Autodesk Inventor part; units mm, degrees
ref_plane "Work Plane1" through (0, 0, -15) normal (0, 0, 1) x (1, 0, 0)
ref_plane "YZ Plane" through (0, 0, 0) normal (1, 0, 0) x (0, 1, 0)
ref_plane "XZ Plane" through (0, 0, 0) normal (0, 1, 0) x (-1, 0, 0)
sketch "Sketch1" plane through (0, 0, 0) normal (0, 0, 1) x (1, 0, 0)
  line L0 (0, 0) -> (25, 0)
  line L1 (25, 0) -> (25, 40)
  line L2 (25, 40) -> (0, 40)
  line L3 (0, 40) -> (0, 0)
  dimension "d1" = 25
  dimension "d2" = 40
  dimension "d3" = 25
extrude "Extrusion1" add sketch "Sketch1" against normal blind 30
sketch "Sketch2" plane through (25, 0, 0) normal (1, 0, 0) x (0, 0, -1)
  line L0 (0, 0) -> (30, 0)
  circle A0 centre (15, 6.56) radius 2.46
extrude "Extrusion2" cut sketch "Sketch2" against normal blind 30
sketch "Sketch3" plane through (0, 0, 0) normal (-1, 0, 0) x (0, 0, 1)
  line L0 (0, 0) -> (-30, 0)
  line L1 (-25.05, 0) -> (-4.95, 0)
  line L2 (-4.95, 0) -> (-4.95, 33.12)
  line L3 (-4.95, 33.12) -> (-25.05, 33.12)
  line L4 (-25.05, 33.12) -> (-25.05, 0)
  dimension "d11" = 20.1
extrude "Extrusion3" cut sketch "Sketch3" against normal blind 20
sketch "Sketch4" plane through (0, 0, 0) normal (0, -1, 0) x (1, 0, 0)
  line L0 (20, -4.95) -> (20, -25.05)
  line L1 (20, -15) -> (25, -15)
  line L2 (25, 0) -> (25, -30)
  line L3 (20, -8.025) -> (25, -8.025)
  line L4 (25, -8.025) -> (25, -21.975)
  line L5 (25, -21.975) -> (20, -21.975)
  line L6 (20, -21.975) -> (20, -8.025)
  line L7 (20, -8.025) -> (25, -21.975) construction
  line L8 (25, -8.025) -> (20, -21.975) construction
  line L9 (25, -12.54) -> (25, -17.46)
  point P0 (0, 0)
  point P1 (22.5, -15)
  dimension "d14" = 13.95
extrude "Extrusion4" add sketch "Sketch4" along normal blind 15
sketch "Sketch5" plane through (20, 0, 0) normal (-1, 0, 0) x (0, 0, 1)
  circle A0 centre (-15, 6.56) radius 2.46
  circle A1 centre (-15, 6.56) radius 4.7025
  circle A2 centre (-15, 6.56) radius 2.46
  circle A3 centre (-15, 6.56) radius 2.46
  point P0 (0, 0)
  dimension "d17" = 9.405
extrude "Extrusion5" cut sketch "Sketch5" against normal blind 2.1
sketch "Sketch6" plane through (25, 0, 0) normal (1, 0, 0) x (0, 0, -1)
  circle A0 centre (15, 6.56) radius 4.7025
  line L0 (15, 6.56) -> (15, 23.56)
  circle A1 centre (15, 23.56) radius 2.46
  point P0 (0, 0)
  dimension "d20" = 17
  dimension "d21" = 4.92
extrude "Extrusion6" cut sketch "Sketch6" against normal blind 10 contours A1
sketch "Sketch7" plane through (20, 0, 0) normal (-1, 0, 0) x (0, 0, 1)
  circle A0 centre (-15, 23.56) radius 2.46
  circle A1 centre (-15, 23.56) radius 4.7025
  point P0 (0, 0)
  dimension "d24" = 9.405
extrude "Extrusion7" cut sketch "Sketch7" against normal blind 2.1
sketch "Sketch9" plane through (25, 0, 0) normal (1, 0, 0) x (0, 0, -1)
  circle A0 centre (15, 6.56) radius 2.46
  circle A1 centre (15, 6.56) radius 2.46
  circle A2 centre (15, 23.56) radius 2.46
  circle A3 centre (15, 23.56) radius 2.46
  line L0 (30, 40) -> (30, 0)
  line L1 (30, 0) -> (30, 40)
  line L2 (30, 40) -> (0, 40)
  line L3 (0, 40) -> (0, 0)
  line L4 (0, 0) -> (8.025, 0)
  line L5 (21.975, 0) -> (21.975, -15)
  line L6 (21.975, -15) -> (8.025, -15)
  line L7 (8.025, -15) -> (8.025, 0)
  line L8 (0, 0) -> (8.025, 0)
  line L9 (21.975, 0) -> (30, 0)
extrude "Extrusion8" add sketch "Sketch9" along normal blind 5
sketch "Sketch10" plane through (0, 40, 0) normal (0, 1, 0) x (1, 0, 0)
  line L0 (0, 30) -> (30, 30)
  line L1 (30, 0) -> (0, 0)
  line L2 (0, 30) -> (30, 30)
  line L3 (30, 30) -> (30, 0)
  line L4 (30, 0) -> (0, 0)
  line L5 (0, 0) -> (0, 30)
extrude "Extrusion9" add sketch "Sketch10" along normal blind 30
sketch "Sketch12" plane through (30, 0, 0) normal (1, 0, 0) x (0, 0, -1)
  circle A0 centre (15, 6.56) radius 2.46
  line L0 (15, 6.56) -> (15, 15.06)
  circle A1 centre (15, 15.06) radius 2.525
  point P0 (0, 0)
  dimension "d31" = 8.5
  dimension "d33" = 5.05
extrude "Extrusion10" cut sketch "Sketch12" against normal blind 30 contours A1
sketch "Sketch14" plane through (0, 0, 0) normal (0, 0, 1) x (1, 0, 0)
  line L0 (30, 70) -> (0, 70)
  line L1 (0, 70) -> (0, 85)
  line L2 (30, 0) -> (30, 70)
  line L3 (30, 122.5) -> (30, 70)
  line L4 (30, 105) -> (30, 100)
  line L5 (-12, 153) -> (15, 153)
  line L6 (-7, 150.5) -> (-12, 153)
  line L7 (-7, 102.5) -> (-12, 100)
  line L8 (-7, 102.5) -> (-2, 126.5)
  line L9 (-2, 126.5) -> (-7, 150.5)
  line L10 (30, 126.5) -> (15, 153)
  line L11 (30, 122.5) -> (30, 126.5)
  line L12 (0, 85) -> (0, 100)
  line L13 (0, 100) -> (-12, 100)
  point P0 (0, 0)
  dimension "d90" = 12
extrude "Extrusion12" add sketch "Sketch14" against normal blind 30
sketch "Sketch15" plane through (0, 0, -25.05) normal (-1, 0, 0) x (0, 0, 1)
  line L0 (0, 33.12) -> (20.1, 33.12)
  line L1 (20.1, 33.12) -> (20.1, 0)
  line L2 (0, 33.12) -> (20.1, 33.12)
  line L3 (20.1, 33.12) -> (20.1, 31.1)
  line L4 (20.1, 31.1) -> (0, 31.1)
  line L5 (0, 31.1) -> (0, 33.12)
  point P0 (25.05, 0)
  dimension "d57" = 2.02
extrude "Extrusion13" add sketch "Sketch15" against normal blind 20
sketch "Sketch25" plane through (0, 0, 0) normal (0, 0, 1) x (1, 0, 0)
  line L0 (0, 100) -> (-12, 100)
  line L1 (0, 100) -> (-12, 100)
  line L2 (-12, 100) -> (-7, 102.5)
  line L3 (-12, 100) -> (-7, 102.5)
  line L4 (-7, 102.5) -> (-2, 126.5)
  line L5 (-7, 102.5) -> (-2, 126.5)
  line L6 (-2, 126.5) -> (-7, 150.5)
  line L7 (-2, 126.5) -> (-7, 150.5)
  line L8 (-7, 150.5) -> (-12, 153)
  line L9 (-7, 150.5) -> (-12, 153)
  line L10 (-12, 153) -> (15, 153)
  line L11 (-12, 153) -> (15, 153)
  line L12 (15, 153) -> (30, 126.5)
  line L13 (15, 153) -> (30, 126.5)
  line L14 (30, 126.5) -> (30, 86.5)
  line L15 (30, 0) -> (30, 126.5)
  line L16 (30, 86.5) -> (0, 86.5)
  line L17 (0, 100) -> (0, 0)
  line L18 (0, 86.5) -> (0, 100)
  dimension "d91" = 40
  dimension "d92" = 30
extrude "Extrusion14" add sketch "Sketch25" along normal blind 30
ref_plane "Work Plane1" through (0, 0, -15) normal (0, 0, 1) x (1, 0, 0)
mirror "Mirror1" about plane through (0, 0, -15) normal (0, 0, 1) of "Extrusion14"
properties part number "rec_b_48mm_x_90mm"
Model file for the job. Use its own axes, mm. A direction names the side the tool comes from. Round coordinates to 2 decimals unless told otherwise and drop trailing zeros. Write each loop counter-clockwise with the first axis right and the second up, starting at its lowest first coordinate (ties: lowest second). Pieces come first, ordered by that corner, then holes. Notation, with made-up numbers: M -9.75,0 L -3.75,0 A21 ccw -3.75,30 Z; hole C 14.25,-12 d5. An arc over 180 degrees is marked long. Put each result on its own line as item: value.
Item 1: Cut at D-D (x = 12). List the corners of the cut face in (y, z), and give its area (3 significant figures).
Responses:
outline: M 0,-30 L 86.5,-30 L 86.5,-60 L 153,-60 L 153,30 L 86.5,30 L 86.5,0 L 0,0 L 0,-4.95 L 31.1,-4.95 L 31.1,-25.05 L 0,-25.05 Z
area: 7,950 mm²
Item 2: Probe L1, parallel to Z at x = 28.25, y = 6.56; L2, parallel to Y at x = 22.75, z = -15 (3 decimals); L3, parallel to Y at x = 21.5, z = -15 (1 decimal). List the from-to ranges inside material, lowest first. Write a range as from..to.
Responses:
L1: -30..-17.46, -12.54..0
L2: -15..4.1, 9.02..12.535, 17.585..21.1, 26.02..139.308
L3: -15..1.9, 11.3..12.5, 17.6..18.9, 28.3..141.5
Item 3: Cut at A-A (x = -5). List the corners of the cut face in (y, z).
Responses:
outline: M 100,-60 L 112.1,-60 L 112.1,30 L 100,30 Z; M 140.9,-60 L 153,-60 L 153,30 L 140.9,30 Z
Item 4: Flat gauge pins, fed straight in: P1, Ø5, axis at x = 24, y = 3.5, coming from the +Z side; P2, Ø24, axis at x = 22, z = 11, coming from the -Y side; P3, Ø4.5, axis at y = 8.5, z = -13, coming from the -X side; P4, Ø3, axis at y = 23.56, z = -15, coming from the +X side. Where does each tip first touch, or does it go through?
Responses:
P1: z = 0
P2: y = 0
P3: x = 20
P4: through
Item 5: Cut at C-C (z = -15). State how many separate pieces and enclosed holes the cut face has, and give its area (3 significant figures).
Responses:
separate pieces: 4
enclosed holes: 0
area: 4,020 mm²
Item 6: Cut at B-B (y = 6.56). List the corners of the cut face in (x, z), and give its area (3 significant figures).
Responses:
outline: M 0,-30 L 30,-30 L 30,-17.46 L 22.1,-17.46 L 22.1,-19.7 L 20,-19.7 L 20,-25.05 L 0,-25.05 Z; M 0,-4.95 L 20,-4.95 L 20,-10.3 L 22.1,-10.3 L 22.1,-12.54 L 30,-12.54 L 30,0 L 0,0 Z
area: 439 mm²
Item 7: Tool access for faces 5 (the flat face through (-4.465, 114.668, -14.37)), 6 (the flat face through (10, 16, -25.05)), 7 (the flat face through (18, 0, -27)), 8 (the cylindrical face through (21.035, 7.973, -10.515)), 9 (the flat face through (15, 0, -3)): list every direction of +Z, -Z, +X, -X, +Y, -Y with a clear straight run to the whole face (end or side of a thin tool).
Responses:
face 5: +Z, -Z, -X
face 6: -X, -Y
face 7: -Z, +X, -X, -Y
face 8: -X
face 9: +Z, +X, -X, -Y
Item 8: Mould opens along Z. For faces 1 (the flat face through (-10, 152, -14)), 2 (the flat face through (25, -8, -8.025)), 3 (the cylindrical face through (21.035, 27.525, -12.472)), 4 (the flat face through (15, 44, -30)) say: +Z half, -Z half, draft (parallel to the pull), parting line (faces both ways), or undercut.
Responses:
face 1: draft
face 2: +Z half
face 3: undercut
face 4: -Z half
